Check sheet for the modelled part. Datum: model origin and axes. Units: mm. Face numbers are marked on the shaded views. A direction names the side the tool comes from. Coordinates: 2 decimals unless noted, no trailing zeros. Order: outer loops, then holes, each group sorted by start corner. A loop starts at its lowest first (then second) coordinate and runs counter-clockwise, first axis right, second up.
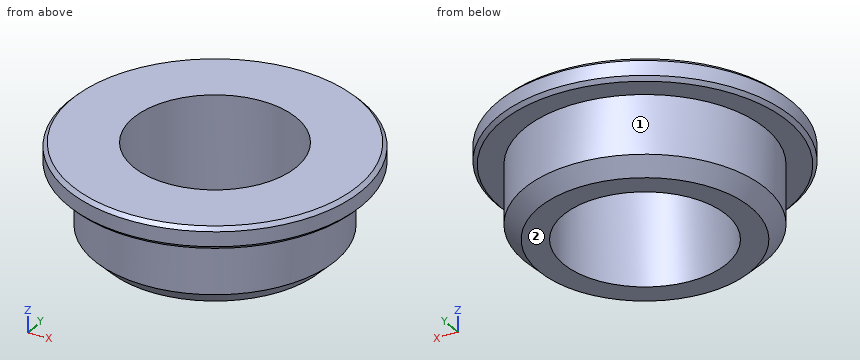
Autodesk Inventor part; units mm, degrees
ref_plane "YZ Plane" through (0, 0, 0) normal (1, 0, 0) x (0, 1, 0)
ref_plane "XZ Plane" through (0, 0, 0) normal (0, 1, 0) x (-1, 0, 0)
ref_plane "XY Plane" through (0, 0, 0) normal (0, 0, 1) x (1, 0, 0)
sketch "スケッチ1" plane through (0, 0, 0) normal (0, 0, 1) x (1, 0, 0)
  circle A0 centre (0, 0) radius 16.4
  dimension "d0" = 32.8
extrude "押し出し1" add sketch "スケッチ1" along normal blind 10
sketch "スケッチ2" plane through (0, 0, 10) normal (0, 0, 1) x (1, 0, 0)
  circle A0 centre (0, 0) radius 16.4
  circle A1 centre (0, 0) radius 20
  dimension "d3" = 40
extrude "押し出し2" add sketch "スケッチ2" along normal blind 3 contours A0 | A1
chamfer "面取り1" distance 2 angle 45 1 edges at (-16.4, 0, 0)
chamfer "面取り2" distance 0.5 angle 45 2 edges at (-20, 0, 13) (-20, 0, 10)
sketch "スケッチ3" plane through (0, 0, 13) normal (0, 0, 1) x (1, 0, 0)
  circle A0 centre (0, 0) radius 19.5
  circle A1 centre (0, 0) radius 11.1
  dimension "d12" = 22.2
extrude "押し出し3" cut sketch "スケッチ3" against normal through all contours A1
properties part number "Print_Parts_P" material "PC/ABS プラスチック"
(1) Cross-section at A-A (y = 0). Enter the section's corners in (x, z).
Filled in:
outline: (-20, 10.5) - (-19.5, 10) - (-16.4, 10) - (-16.4, 2) - (-14.4, 0) - (-11.1, 0) - (-11.1, 13) - (-19.5, 13) - (-20, 12.5) - close; (11.1, 0) - (14.4, 0) - (16.4, 2) - (16.4, 10) - (19.5, 10) - (20, 10.5) - (20, 12.5) - (19.5, 13) - (11.1, 13) - close
(2) Tool access check on the marked faces 1 and 2. Record the directions out of +Z, -Z, +X, -X, +Y, -Y that give a thin tool (end or side, any length) a straight path to the whole face; none if there is none.
Filled in:
face 1: -Z
face 2: -Z, +X, -X, +Y, -Y
(3) Thickness scan on probe 1 along Y at (x, z) = (0, 5); probe 2 along X at (y, z) = (0.5, 5.25); probe 3 along Z at (x, y) = (-14, -12). Record the ranges inside material, lowest first.
Filled in:
probe 1: y = -16.4 to -11.1, 11.1 to 16.4
probe 2: x = -16.39 to -11.09, 11.09 to 16.39
probe 3: z = 10 to 13
(4) Cross-section at C-C (z = 5). Enter the section's corners in (x, y), and give its area (3 significant figures).
Filled in:
outline: circle Ø32.8 at (0, 0); hole circle Ø22.2 at (0, 0)
area: 458 mm2
(5) Go/stop test with flat-tipped pins: P1, Ø2, axis at x = 16, y = -8, coming from the -Z side; P2, Ø4, axis at x = 2, z = 9.5, coming from the +Y side; P3, Ø1, axis at x = -6, z = 7, coming from the +Y side. Record where each tip stops, or that it passes through.
Filled in:
P1: stops at z = 10
P2: stops at y = 20
P3: stops at y = 15.45
